Drawing for the job (mm, zero at the part's lowest x, y, z). A direction names the side the tool comes from. Coordinates: 2 decimals unless noted, no trailing zeros. Order: outer loops, then holes, each group sorted by start corner. A loop starts at its lowest first (then second) coordinate and runs counter-clockwise, first axis right, second up.
1) Cut at B-B (z = 19.5). List the corners of the cut face in (x, y).
2) Cut at C-C (y = 2.75). List the corners of the cut face in (x, z), and give its area (3 significant figures).
3) Cut at A-A (x = 4.8). List the corners of the cut face in (y, z).
4) Tool access for the marked faces 4 and 5: list every direction of +Z, -Z, +X, -X, +Y, -Y with a clear straight run to the whole face (end or side of a thin tool).
5) Wall check: L1, parallel to Z at x = 4.8, y = 0.4; L2, parallel to Z at x = 15.25, y = 3.75; L3, parallel to Y at x = 9, z = 13.75. Give the ranges that are in metal, low to high.
6) Pin check, flat tips, straight feed: pin 1 Ø1 at (x, z) = (12, 9.5) entering from +Y; pin 2 Ø1 at (y, z) = (1, 9.5) entering from +X. Stop position of each tip, or through.
7) Mould opens along Z. For the marked faces 1, 2 and 3 say: +Z half, -Z half, draft (parallel to the pull), parting line (faces both ways), or undercut.
8) Cut at D-D (z = 2.5). List the corners of the cut face in (x, y), and give its area (3 significant figures).
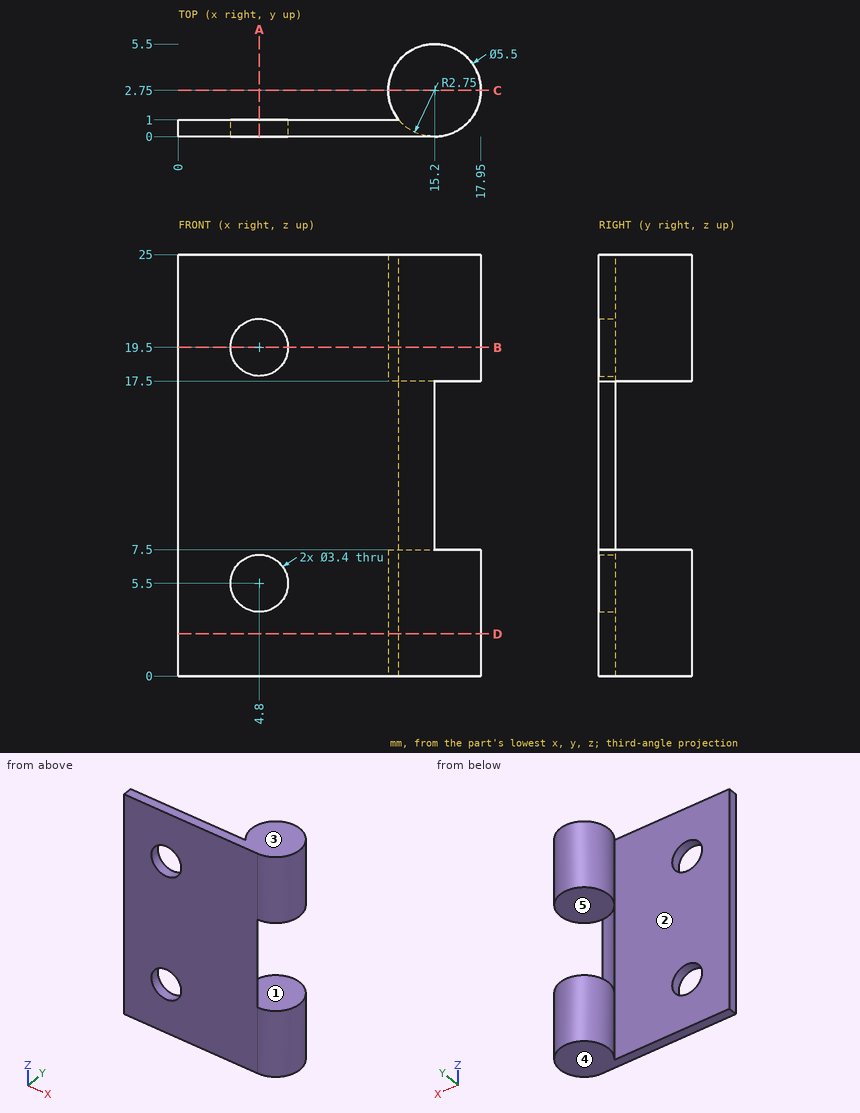
Geometry check:
1. outline: (0, 0) - (3.1, 0) - (3.1, 1) - (0, 1) - close; (6.5, 0) - (15.2, 0) arc R2.75 ccw (long way) to (13.08, 1) - (6.5, 1) - close
2. outline: (12.45, 0) - (17.95, 0) - (17.95, 7.5) - (12.45, 7.5) - close; (12.45, 17.5) - (17.95, 17.5) - (17.95, 25) - (12.45, 25) - close
2. area: 82.5 mm2
3. outline: (0, 0) - (1, 0) - (1, 3.8) - (0, 3.8) - close; (0, 7.2) - (1, 7.2) - (1, 17.8) - (0, 17.8) - close; (0, 21.2) - (1, 21.2) - (1, 25) - (0, 25) - close
4. face 4: -Z, +X, -X, +Y, -Y
4. face 5: +X, +Y
5. L1: z = 0 to 3.8, 7.2 to 17.8, 21.2 to 25
5. L2: z = 0 to 7.5, 17.5 to 25
5. L3: y = 0 to 1
6. pin 1: stops at y = 1
6. pin 2: stops at x = 13.62
7. face 1: undercut
7. face 2: draft
7. face 3: +Z half
8. outline: (0, 0) - (15.2, 0) arc R2.75 ccw (long way) to (13.08, 1) - (0, 1) - close
8. area: 37.5 mm2
